```python
from build123d import *

# Parameters (mm, degrees)
SKETCH1_W           = 55
SKETCH1_H           = 55
BOSS_EXTRUDE1_DEPTH = 10
BOSS_EXTRUDE3_DEPTH = 15
SKETCH3_W           = 55
SKETCH3_H           = 55
SKETCH3_W_2         = 40.6
SKETCH3_H_2         = 40
BOSS_EXTRUDE5_DEPTH = 15
SKETCH7_W           = 12
SKETCH7_H           = 24.88370491
CUT_EXTRUDE3_DEPTH  = 30
SKETCH8_R           = 2
CUT_EXTRUDE4_DEPTH  = 7
SKETCH9_R           = 2
CUT_EXTRUDE5_DEPTH  = 7


with BuildPart() as part:
    # Sketch1 → Boss-Extrude1 (new body)
    with BuildSketch(Plane(origin=(0, 0, 0), x_dir=(1, 0, 0), z_dir=(0, 1, 0))):
        with Locations((-27.5, -27.5)):
            Rectangle(SKETCH1_W, SKETCH1_H)
    extrude(amount=BOSS_EXTRUDE1_DEPTH)

    # Sketch2 → Boss-Extrude3 (add)
    with BuildSketch(Plane(origin=(0, 10, 0), x_dir=(1, 0, 0), z_dir=(0, 1, 0))):
        Polygon((-45.31629509, -17.267409819), (-43.11629509, -17.267409819), (-43.11629509, -14.767409819), (-41.61629509, -14.767409819), (-39, -17.38370491), (-39, -22.88370491), (-41.61629509, -25.5), (-43.11629509, -25.5), (-43.11629509, -23.3), (-45.31629509, -23.3), align=None)
        Polygon((-6.88370491, -23.3), (-4.68370491, -23.3), (-4.68370491, -17.267409819), (-6.88370491, -17.267409819), (-6.88370491, -14.767409819), (-8.38370491, -14.767409819), (-11, -17.38370491), (-11, -22.88370491), (-8.38370491, -25.5), (-6.88370491, -25.5), align=None)
        Polygon((-43.11629509, -36.7), (-45.31629509, -36.7), (-45.31629509, -42.732590181), (-43.11629509, -42.732590181), (-43.11629509, -45.232590181), (-41.61629509, -45.232590181), (-39, -42.61629509), (-39, -37.11629509), (-41.61629509, -34.5), (-43.11629509, -34.5), align=None)
        Polygon((-6.88370491, -34.5), (-6.88370491, -36.7), (-4.68370491, -36.7), (-4.68370491, -42.732590181), (-6.88370491, -42.732590181), (-6.88370491, -45.232590181), (-8.38370491, -45.232590181), (-11, -42.61629509), (-11, -37.11629509), (-8.38370491, -34.5), align=None)
    extrude(amount=BOSS_EXTRUDE3_DEPTH)

    # Sketch3 → Boss-Extrude5 (add)
    with BuildSketch(Plane(origin=(0, 10, 0), x_dir=(1, 0, 0), z_dir=(0, 1, 0))):
        with Locations((-27.5, -27.5)):
            Rectangle(SKETCH3_W, SKETCH3_H)
        with Locations((-25, -30)):
            Rectangle(SKETCH3_W_2, SKETCH3_H_2, mode=Mode.SUBTRACT)
    extrude(amount=BOSS_EXTRUDE5_DEPTH)

    # Sketch7 → Cut-Extrude3 (cut)
    with BuildSketch(Plane(origin=(0, 25, 0), x_dir=(1, 0, 0), z_dir=(0, 1, 0))):
        with Locations((-25, -12.441852455)):
            Rectangle(SKETCH7_W, SKETCH7_H)
    extrude(amount=-CUT_EXTRUDE3_DEPTH, mode=Mode.SUBTRACT)

    # Sketch8 → Cut-Extrude4 (cut)
    with BuildSketch(Plane(origin=(0, 0, 0), x_dir=(-1, 0, 0), z_dir=(0, 0, -1))):
        with Locations((50, 9)):
            Circle(SKETCH8_R)
    extrude(amount=-CUT_EXTRUDE4_DEPTH, mode=Mode.SUBTRACT)

    # Sketch9 → Cut-Extrude5 (cut)
    with BuildSketch(Plane.XZ):
        with Locations(Location((-40, 42, 0), (0, 0, 270))):
            Circle(SKETCH9_R)
        with Locations(Location((-50, 42, 0), (0, 0, 270))):
            Circle(SKETCH9_R)
    extrude(amount=-CUT_EXTRUDE5_DEPTH, mode=Mode.SUBTRACT)


solid = part.part
```
The listing builds one solid part. Answer for the finished solid, in the listing's coordinates (mm). A direction names the side the tool comes from. Coordinates: 2 decimals unless noted, no trailing zeros. Write each loop counter-clockwise with the first axis right and the second up, starting at its lowest first coordinate (ties: lowest second). Pieces come first, ordered by that corner, then holes. Notation, with made-up numbers: (-35.5, 14) - (-28.5, 14) arc R25 ccw to (-28.5, 42) - close; hole circle Ø7 at (89, -2). An arc over 180 degrees is marked (long way). One line per item, written item: value.
1) Find section A-A (y = 4.5). Give the vertices of the cut face in (x, z), and give its area (3 significant figures).
Geometry check:
outline: (-55, 0) - (-31, 0) - (-31, 24.88) - (-19, 24.88) - (-19, 0) - (0, 0) - (0, 55) - (-55, 55) - close; hole circle Ø4 at (-50, 42); hole circle Ø4 at (-40, 42)
area: 2,700 mm2
2) A tool of negligible diameter and unlimited length cuts with its end or side. For faces 1 (the flat face through (-11, 17, 40)), 2 (the flat face through (-28, 0, 27)), 3 (the cylindrical face through (-52, 3, 42)), from which of +Z, -Z, +X, -X, +Y, -Y can it reach the whole face along a straight path? Write none if from no direction.
Geometry check:
face 1: +Y
face 2: +Z, -Z, +X, -X, -Y
face 3: -Y
3) Find section C-C (x = -40). Give the vertices of the cut face in (y, z), and give its area (3 significant figures).
Geometry check:
outline: (0, 0) - (25, 0) - (25, 10) - (10, 10) - (10, 16.38) - (25, 16.38) - (25, 23.88) - (10, 23.88) - (10, 36.12) - (25, 36.12) - (25, 43.62) - (10, 43.62) - (10, 50) - (25, 50) - (25, 55) - (0, 55) - (0, 44) - (7, 44) - (7, 40) - (0, 40) - close
area: 972 mm2
4) Consider line 1 along X through (y, z) = (1.75, 42); line 2 along X through (y, z) = (2.5, 14.5); line 3 along Z through (x, y) = (-8, 18.75). Determine where each line is inside the solid, lowest interval first. Write a range as from..to.
Geometry check:
line 1: x = -55..-52, -48..-42, -38..0
line 2: x = -55..-31, -19..0
line 3: z = 0..10, 14.77..25.5, 34.5..45.23, 50..55
5) Find section B-B (z = 32). Give the vertices of the cut face in (x, y).
Geometry check:
outline: (-55, 0) - (0, 0) - (0, 25) - (-4.7, 25) - (-4.7, 10) - (-45.3, 10) - (-45.3, 25) - (-55, 25) - close
6) Find section D-D (y = 9). Give the vertices of the cut face in (x, z).
Geometry check:
outline: (-55, 0) - (-52, 0) - (-52, 7) - (-48, 7) - (-48, 0) - (-31, 0) - (-31, 24.88) - (-19, 24.88) - (-19, 0) - (0, 0) - (0, 55) - (-55, 55) - close
7) Each of these flat-tipped pins is pushed along its axis until it touches: pin 1 Ø3 at (x, y) = (-24.5, 5.5) entering from -Z; pin 2 Ø1.2 at (x, y) = (-50.5, 8.5) entering from -Z; pin 3 Ø8 at (x, z) = (-34, 41.5) entering from +Y. Where does it stop, or does it pass through?
Geometry check:
pin 1: stops at z = 24.88
pin 2: stops at z = 7
pin 3: stops at y = 10
